Part model, mm, in its own coordinate system. Face numbers are marked on the shaded views. A direction names the side the tool comes from. Give positions to 0.01 mm unless a question says otherwise; leave off trailing zeros. Write each loop counter-clockwise with the first axis right and the second up, starting at its lowest first coordinate (ties: lowest second). Pieces come first, ordered by that corner, then holes. Notation, with made-up numbers: M 74.25,19.5 L 82.25,19.5 A29 cw 82.25,46.5 Z; hole C 71.25,10 d8. An arc over 180 degrees is marked long. Answer as CSV lines item,"result". Start each with the question number.
1) Slice it at C-C, the plane x = -6.75. Give the cut face in (y, z), plus the area to 3 significant figures.
2) Mould opens along X. For the marked faces 6, 7 and 8 say: pulls with the +X half, pulls with the -X half, needs draft (parallel to the pull), parting line crosses it, or undercut.
3) Slice it at D-D, the plane z = 4.25. Give the cut face in (x, y).
4) Tool access for the marked faces 1, 2, 3, 4 and 5: list every direction of +Z, -Z, +X, -X, +Y, -Y with a clear straight run to the whole face (end or side of a thin tool).
5) Slice it at A-A, the plane z = 3. Give the cut face in (x, y), plus the area to 3 significant figures.
6) Wall check: line 1 along X through (y, z) = (-0.5, 3); line 2 along Z through (x, y) = (7, -1.5); line 3 along X through (y, z) = (1.25, 1.75). Give the ranges that are in metal, low to high. Write a range as from..to.
7) Slice it at B-B, the plane y = 5.5. Give the cut face in (x, z).
8) Pin check, flat tips, straight feed: pin 1 Ø1.5 at (y, z) = (-2, 3.5) entering from -X; pin 2 Ø2 at (x, z) = (-1.5, 1) entering from +Y; pin 3 Ø3 at (x, z) = (3, 1) entering from -Y; pin 4 Ø10 at (x, y) = (-2.5, -2.5) entering from -Z. Stop position of each tip, or through.
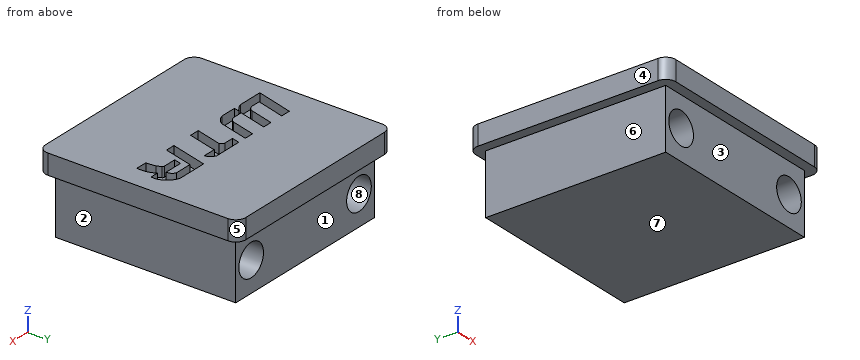
```python
from build123d import *

# Parameters (mm, degrees)
SKETCH_1_W          = 18
SKETCH_1_H          = 18
EXTRUDE_1_DEPTH     = 6
SKETCH_2_R          = 1.6
CUT_EXTRUDE_1_DEPTH = 19
SKETCH_3_W          = 20
SKETCH_3_H          = 20
EXTRUDE_2_DEPTH     = 2
FILLET_1_R          = 1
CUT_EXTRUDE_2_DEPTH = 1


with BuildPart() as part:
    # 草图1 → 凸台-拉伸1 (new body)
    with BuildSketch(Plane.XY):
        Rectangle(SKETCH_1_W, SKETCH_1_H)
    extrude(amount=EXTRUDE_1_DEPTH)

    # 草图2 → 切除-拉伸1 (cut, through all)
    with BuildSketch(Plane(origin=(0, 9, 0), x_dir=(1, 0, 0), z_dir=(0, 1, 0))):
        with Locations((-7, -3)):
            Circle(SKETCH_2_R)
        with Locations((7, -3)):
            Circle(SKETCH_2_R)
    extrude(amount=-CUT_EXTRUDE_1_DEPTH, mode=Mode.SUBTRACT)

    # 草图3 → 凸台-拉伸2 (add)
    with BuildSketch(Plane.XY.offset(6)):
        Rectangle(SKETCH_3_W, SKETCH_3_H)
    extrude(amount=EXTRUDE_2_DEPTH)

    # 圆角1
    fillet_1_edges = [part.edges().sort_by_distance(p)[0] for p in [
        (10, -10, 7),
        (10, 10, 7),
        (-10, 10, 7),
        (-10, -10, 7),
    ]]
    fillet(fillet_1_edges, radius=FILLET_1_R)

    # 草图5 → 切除-拉伸2 (cut)
    with BuildSketch(Plane.XY.offset(8)):
        with BuildLine():
            Line((-7.204561004, 1.879394949), (-8.234522443, -1.859506165))
            Line((-8.234522443, -1.859506165), (-5.723109619, -1.859506165))
            ThreePointArc((-5.723109619, -1.859506165), (-5.218538697, -1.632457047), (-4.78861912, -1.284157931))
            Line((-4.78861912, -1.284157931), (-4.947111275, -1.859506165))
            Line((-4.947111275, -1.859506165), (-3.352787404, -1.859506165))
            ThreePointArc((-3.352787404, -1.859506165), (-2.759972983, -1.585355224), (-2.30360072, -1.118116491))
            Line((-2.30360072, -1.118116491), (-1.497804292, 1.879394949))
            Line((-1.497804292, 1.879394949), (-2.436323584, 1.879394949))
            Line((-2.436323584, 1.879394949), (-3.079504637, -0.513197642))
            ThreePointArc((-3.079504637, -0.513197642), (-3.32542599, -0.827982147), (-3.696433402, -0.976036515))
            Line((-3.696433402, -0.976036515), (-4.666789972, -0.976036515))
            Line((-4.666789972, -0.976036515), (-3.880199418, 1.879394949))
            Line((-3.880199418, 1.879394949), (-4.81871871, 1.879394949))
            Line((-4.81871871, 1.879394949), (-5.477810253, -0.513197642))
            ThreePointArc((-5.477810253, -0.513197642), (-5.7047457, -0.820725721), (-6.053961641, -0.976036515))
            Line((-6.053961641, -0.976036515), (-7.003517302, -0.976036515))
            Line((-7.003517302, -0.976036515), (-6.216926747, 1.879394949))
            Line((-6.216926747, 1.879394949), (-7.204561004, 1.879394949))
        make_face()
        with BuildLine():
            Line((-0.857127264, 1.088853082), (-0.644612375, 1.879394949))
            Line((-0.644612375, 1.879394949), (2.196209614, 1.879394949))
            ThreePointArc((2.196209614, 1.879394949), (2.612575491, 1.570775142), (2.803252851, 1.088853082))
            Line((2.803252851, 1.088853082), (1.498562909, 1.088853082))
            Line((1.498562909, 1.088853082), (1.498562909, 0.920146657))
            Line((1.498562909, 0.920146657), (0.751331627, -1.859506165))
            Line((0.751331627, -1.859506165), (-0.236975463, -1.859506165))
            Line((-0.236975463, -1.859506165), (0.463990432, 0.748042361))
            ThreePointArc((0.463990432, 0.748042361), (0.35056842, 0.970657535), (0.130450539, 1.088853082))
            Line((0.130450539, 1.088853082), (-0.857127264, 1.088853082))
        make_face()
        with BuildLine():
            Line((3.92496477, 1.879394949), (2.919866632, -1.859506165))
            Line((2.919866632, -1.859506165), (3.879786702, -1.859506165))
            Line((3.879786702, -1.859506165), (4.67236995, 1.088853082))
            Line((4.67236995, 1.088853082), (6.439189541, 1.088853082))
            ThreePointArc((6.439189541, 1.088853082), (6.74191311, 0.79302609), (6.831437365, 0.379334689))
            Line((6.831437365, 0.379334689), (4.973337874, 0.379334689))
            Line((4.973337874, 0.379334689), (4.777076341, -0.350745725))
            Line((4.777076341, -0.350745725), (6.123295998, -0.350745725))
            ThreePointArc((6.123295998, -0.350745725), (6.221884558, -0.372626448), (6.288711068, -0.448340962))
            Line((6.288711068, -0.448340962), (6.481965147, -0.894824524))
            ThreePointArc((6.481965147, -0.894824524), (6.543334906, -1.375731382), (6.574951556, -1.859506165))
            Line((6.574951556, -1.859506165), (7.717356009, -1.859506165))
            ThreePointArc((7.717356009, -1.859506165), (7.71253802, -0.938991532), (7.378394237, -0.081251283))
            Line((7.378394237, -0.081251283), (8.199786702, -0.081251283))
            ThreePointArc((8.199786702, -0.081251283), (7.934816182, 1.144935193), (6.917805112, 1.879394949))
            Line((6.917805112, 1.879394949), (3.92496477, 1.879394949))
        make_face()
    extrude(amount=-CUT_EXTRUDE_2_DEPTH, mode=Mode.SUBTRACT)


solid = part.part
```
Found:
1,outline,"M -10,6 L -9,6 L -9,4.58 L 9,4.58 L 9,6 L 10,6 L 10,8 L 1.88,8 L 1.88,7 L -0.06,7 L -0.06,8 L -0.98,8 L -0.98,7 L -1.86,7 L -1.86,8 L -10,8 Z; M -9,0 L 9,0 L 9,1.42 L -9,1.42 Z"
1,area,"88.3 mm²"
2,face 6,"pulls with the -X half"
2,face 7,"needs draft"
2,face 8,"undercut"
3,outline,"M -9,-9 L -8,-9 L -8,9 L -9,9 Z; M -6,-9 L 6,-9 L 6,9 L -6,9 Z; M 8,-9 L 9,-9 L 9,9 L 8,9 Z"
4,face 1,"-Z, +X, -X, +Y"
4,face 2,"-Z, +X, +Y, -Y"
4,face 3,"-Z, +X, -X, -Y"
4,face 4,"+Z, -Z, -X, +Y, -Y"
4,face 5,"+Z, -Z, +X, +Y"
5,outline,"M -9,-9 L -8.6,-9 L -8.6,9 L -9,9 Z; M -5.4,-9 L 5.4,-9 L 5.4,9 L -5.4,9 Z; M 8.6,-9 L 9,-9 L 9,9 L 8.6,9 Z"
5,area,"209 mm²"
6,line 1,"-9..-8.6, -5.4..5.4, 8.6..9"
6,line 2,"0..1.4, 4.6..7"
6,line 3,"-9..-8, -6..6, 8..9"
7,outline,"M -10,6 L -9,6 L -9,0 L 9,0 L 9,6 L 10,6 L 10,8 L -10,8 Z; hole C -7,3 d3.2; hole C 7,3 d3.2"
8,pin 1,"x = -9"
8,pin 2,"y = 9"
8,pin 3,"y = -9"
8,pin 4,"z = 0"
